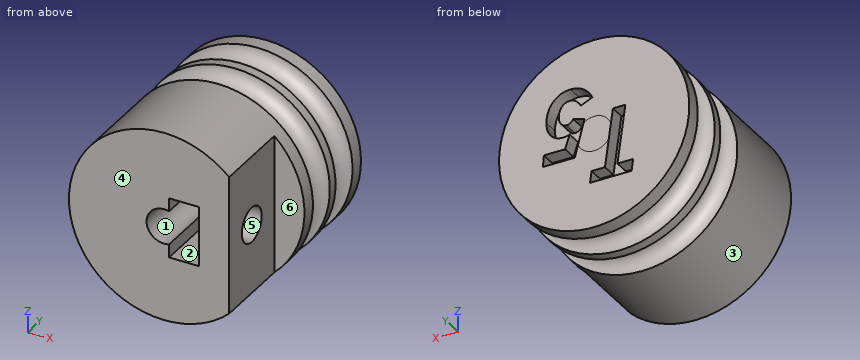
from build123d import *

# Parameters (mm, degrees)
SKETCH1_R               = 9.5
SKETCH1_R_2             = 1.75
BOSS_EXTRUDE1_DEPTH     = 18
SKETCH2_R               = 1.5
CUT_EXTRUDE1_DEPTH      = 23.461077445
CUT_EXTRUDE1_DEPTH_BACK = 23.461077445
SKETCH3_W               = 3
SKETCH3_H               = 8
SKETCH4_W               = 3
SKETCH4_H               = 6
CUT_EXTRUDE2_DEPTH      = 8
CUT_EXTRUDE3_REACH      = 27.889
SKETCH5_R               = 1.75
BOSS_EXTRUDE2_START     = -8.5
SKETCH6_R               = 1.75
BOSS_EXTRUDE2_DEPTH     = 8.5
CUT_EXTRUDE4_DEPTH      = 1.5


with BuildPart() as part:
    # Sketch1 → Boss-Extrude1 (new body)
    with BuildSketch(Plane(origin=(0, 0, 0), x_dir=(1, 0, 0), z_dir=(0, 1, 0))):
        with Locations(Location((0, 0, 0), (0, 0, 270))):
            Circle(SKETCH1_R)
        with Locations(Location((0, 0, 0), (0, 0, 270))):
            Circle(SKETCH1_R_2, mode=Mode.SUBTRACT)
    extrude(amount=BOSS_EXTRUDE1_DEPTH)

    # Sketch2 → Cut-Revolve1 (revolve, cut)
    with BuildSketch(Plane(origin=(0, 0, 0), x_dir=(0, 0, -1), z_dir=(1, 0, 0)), mode=Mode.PRIVATE) as cut_revolve1_sk:
        with Locations((-9.5, 15)):
            Circle(SKETCH2_R)
        with Locations((-9.5, 11)):
            Circle(SKETCH2_R)
    revolve(cut_revolve1_sk.sketch.rotate(Axis((0, 18, 0), (0, -1, 0)), 180), axis=Axis((0, 18, 0), (0, -1, 0)), mode=Mode.SUBTRACT)

    # Sketch3 → Cut-Extrude1 (cut, two sides: drawn at the far end of the back side and taken through both)
    with BuildSketch(Plane.XY.offset(-CUT_EXTRUDE1_DEPTH_BACK)):
        with Locations((8, 4)):
            Rectangle(SKETCH3_W, SKETCH3_H)
    extrude(amount=CUT_EXTRUDE1_DEPTH + CUT_EXTRUDE1_DEPTH_BACK, mode=Mode.SUBTRACT)

    # Sketch4 → Cut-Extrude2 (cut)
    with BuildSketch(Plane.XZ):
        with Locations((2, 0)):
            Rectangle(SKETCH4_W, SKETCH4_H)
    extrude(amount=-CUT_EXTRUDE2_DEPTH, mode=Mode.SUBTRACT)

    # Sketch5 → Cut-Extrude3 (cut, up to next)
    with BuildSketch(Plane(origin=(6.5, 0, 0), x_dir=(0, 0, -1), z_dir=(1, 0, 0)), mode=Mode.PRIVATE) as cut_extrude3_sk1:
        with Locations((0, 4)):
            Circle(SKETCH5_R)
    cut_extrude3_tool1 = extrude(cut_extrude3_sk1.sketch, amount=-CUT_EXTRUDE3_REACH, mode=Mode.PRIVATE) & part.part
    add(cut_extrude3_tool1.solids().sort_by_distance((6.5, 4, 0))[0], mode=Mode.SUBTRACT)

    # Sketch6 → Boss-Extrude2 (add)
    with BuildSketch(Plane(origin=(0, 18, 0), x_dir=(1, 0, 0), z_dir=(0, 1, 0)).offset(BOSS_EXTRUDE2_START)):
        with Locations(Location((0, 0, 0), (0, 0, 73.398450401))):
            Circle(SKETCH6_R)
    extrude(amount=BOSS_EXTRUDE2_DEPTH)

    # Sketch7 → Cut-Extrude4 (cut)
    with BuildSketch(Plane(origin=(0, 18, 0), x_dir=(1, 0, 0), z_dir=(0, 1, 0))):
        Polygon((-3.735416667, 4.879166667), (0.409722222, 4.879166667), (0.260894097, 3.732638889), (-1.078559028, 3.732638889), (-1.873687066, -2), (-3.118055556, -2), (-2.324305556, 3.732638889), (-3.893891059, 3.732638889), align=None)
        with BuildLine():
            Line((1.93063151, 1.879166667), (5.115277778, 1.879166667))
            Line((5.115277778, 1.879166667), (5.027083333, 0.732638889))
            Line((5.027083333, 0.732638889), (2.899392361, 0.732638889))
            Line((2.899392361, 0.732638889), (2.447395833, -0.634375))
            add(Edge.make_bspline(
                [(2.447395833, -0.634375), (2.496594075, -0.613896402), (2.595019861, -0.57292701), (2.749839769, -0.532892585), (2.908139813, -0.506658512), (3.015040488, -0.503615987), (3.068891059, -0.502083333)],
                knots=[0, 0, 0, 0, 0.998112439, 1.996819346, 2.990909824, 4, 4, 4, 4], degree=3))
            add(Edge.make_bspline(
                [(3.068891059, -0.502083333), (3.130977849, -0.503710927), (3.252390467, -0.506893737), (3.430147714, -0.530676662), (3.598897739, -0.570188022), (3.758037558, -0.627264893), (3.908251801, -0.698872885), (4.047892395, -0.787903157), (4.178629893, -0.892282921), (4.299407696, -1.011738133), (4.408795358, -1.145923516), (4.504121795, -1.293773987), (4.584127105, -1.455328827), (4.650907598, -1.628980167), (4.699239379, -1.817024844), (4.736887191, -2.016677617), (4.75910168, -2.230101729), (4.761345538, -2.376622611), (4.7625, -2.452007378)],
                knots=[0, 0, 0, 0, 1.020720285, 1.996049746, 2.943245614, 3.865445419, 4.770849874, 5.674014514, 6.582344456, 7.517049549, 8.461983903, 9.42367584, 10.403295435, 11.421749409, 12.477096939, 13.591170916, 14.760661157, 16, 16, 16, 16], degree=3))
            add(Edge.make_bspline(
                [(4.7625, -2.452007378), (4.760331263, -2.551305248), (4.756082769, -2.745827008), (4.724357481, -3.030366667), (4.670434408, -3.299932267), (4.596788587, -3.55576096), (4.497839346, -3.795403814), (4.381045078, -4.022055988), (4.240535383, -4.23285879), (4.079959926, -4.426863528), (3.90500901, -4.6032865), (3.715999291, -4.755276836), (3.51825895, -4.886229848), (3.309156679, -4.99341577), (3.088438962, -5.074038184), (2.858442877, -5.134443243), (2.617463381, -5.168719531), (2.453470724, -5.173806613), (2.370225694, -5.176388889)],
                knots=[0, 0, 0, 0, 1.173543811, 2.298939634, 3.378629864, 4.419763593, 5.440091566, 6.438176937, 7.429014836, 8.427971092, 9.41078854, 10.360474936, 11.289592146, 12.209863076, 13.130646371, 14.061665239, 15.016073429, 16, 16, 16, 16], degree=3))
            add(Edge.make_bspline(
                [(2.370225694, -5.176388889), (2.310933889, -5.175336104), (2.193952372, -5.173258982), (2.020726741, -5.156555087), (1.852671583, -5.127655453), (1.689527041, -5.086994539), (1.530531877, -5.038216677), (1.376964542, -4.976019014), (1.229625203, -4.900480546), (1.08541527, -4.817015387), (0.94797473, -4.720741688), (0.817898945, -4.612055658), (0.693643574, -4.493656656), (0.576265412, -4.363698122), (0.466116126, -4.222246293), (0.360964906, -4.071122574), (0.264514937, -3.907473589), (0.206115245, -3.793152274), (0.176388889, -3.734960938)],
                knots=[0, 0, 0, 0, 1.022859238, 2.018080294, 2.999190336, 3.962207893, 4.917235095, 5.866490093, 6.816373485, 7.771926692, 8.739336783, 9.707395925, 10.693964512, 11.698357727, 12.725720478, 13.785346591, 14.8727068, 16, 16, 16, 16], degree=3))
            Line((0.176388889, -3.734960938), (1.318782552, -3.225086806))
            add(Edge.make_bspline(
                [(1.318782552, -3.225086806), (1.366983822, -3.296490214), (1.457415836, -3.430452538), (1.598648511, -3.608942531), (1.738402882, -3.749836535), (1.87577747, -3.85858293), (2.016355711, -3.936444461), (2.160759687, -3.990581364), (2.311349194, -4.023320871), (2.413704476, -4.027668904), (2.46531033, -4.029861111)],
                knots=[0, 0, 0, 0, 1.407698414, 2.641030095, 3.71326683, 4.644229953, 5.494388505, 6.328183133, 7.157097367, 8, 8, 8, 8], degree=3))
            add(Edge.make_bspline(
                [(2.46531033, -4.029861111), (2.502597477, -4.028960648), (2.576241743, -4.027182182), (2.684301906, -4.008243163), (2.787874215, -3.97960222), (2.886816155, -3.939640908), (2.979376072, -3.886543817), (3.067364075, -3.822476619), (3.149686009, -3.745907333), (3.2282627, -3.660042601), (3.298101555, -3.562969472), (3.360585167, -3.458803462), (3.411342282, -3.34552927), (3.454177874, -3.225850289), (3.487464002, -3.098113353), (3.509883951, -2.962938195), (3.526380141, -2.82034566), (3.527303997, -2.722613415), (3.527777778, -2.67249349)],
                knots=[0, 0, 0, 0, 0.927075282, 1.831027126, 2.721359743, 3.598085148, 4.478603181, 5.370329063, 6.300781167, 7.271983059, 8.262041119, 9.271703604, 10.289679922, 11.345465186, 12.432354444, 13.569366541, 14.753500788, 16, 16, 16, 16], degree=3))
            add(Edge.make_bspline(
                [(3.527777778, -2.67249349), (3.525364071, -2.599249545), (3.520736664, -2.45883084), (3.479231749, -2.258812343), (3.4090829, -2.080955219), (3.310983371, -1.92926026), (3.194562907, -1.805997587), (3.06438106, -1.714608894), (2.920185823, -1.658694036), (2.819485773, -1.652001198), (2.768478733, -1.648611111)],
                knots=[0, 0, 0, 0, 1.239981349, 2.377214621, 3.442410989, 4.461421974, 5.419299017, 6.29797895, 7.137884662, 8, 8, 8, 8], degree=3))
            add(Edge.make_bspline(
                [(2.768478733, -1.648611111), (2.733962981, -1.650076188), (2.665766285, -1.652970908), (2.565430302, -1.671769102), (2.471751626, -1.70770096), (2.381470388, -1.752665642), (2.299031841, -1.814661474), (2.221082072, -1.888742142), (2.147448466, -1.975747239), (2.105339675, -2.041728663), (2.08359375, -2.075802951)],
                knots=[0, 0, 0, 0, 0.978206346, 1.932753505, 2.875607702, 3.812696253, 4.78098368, 5.784402359, 6.855815662, 8, 8, 8, 8], degree=3))
            Line((2.08359375, -2.075802951), (0.970138889, -1.745073785))
            Line((0.970138889, -1.745073785), (1.93063151, 1.879166667))
        make_face()
    extrude(amount=-CUT_EXTRUDE4_DEPTH, mode=Mode.SUBTRACT)


solid = part.part
Geometry check sheet. Reference: the model listing, model coordinates, mm. Face numbers are marked on the shaded views. A direction names the side the tool comes from. Give positions to 0.01 mm unless a question says otherwise; leave off trailing zeros. Loops run counter-clockwise (first coordinate to the right, second up) from the corner with the lowest first, then second, coordinate; pieces in that order, holes last. Notation, with made-up numbers: M -7.5,65 L 3.5,65 A30 cw 3.5,89 Z; hole C 78,29 d10. An arc over 180 degrees is marked long. Answer as a JSON object with one key per item and string values. Group by question number.
Item 1: Material ranges on L1, parallel to Z at x = 0, y = 3; L2, parallel to Y at x = 4.1, z = 0; L3, parallel to Y at x = 5.25, z = 7, recorded low to high.
Item 2: Gauge pin test, flat ends, axial feed: pin 1 (2.5 mm diameter, centred on y = 6, z = 1.5, fed in from +X); pin 2 (0.8 mm diameter, centred on x = -1.5, y = 17.5, fed in from +Z); pin 3 (1 mm diameter, centred on x = 3.5, y = 5, fed in from +Z). Record the tip position at first contact, or that the pin passes through.
Item 3: Sectioned sample at A-A on y = 7. Record the boundary of the cut face in (x, z).
Item 4: Sectioned sample at C-C on y = 4. Record the boundary of the cut face in (x, z).
Item 5: Mould release check, pull along X, two halves, no side actions. Record for the marked faces 1, 2, 3 and 4: pulls with the +X half, pulls with the -X half, needs draft (parallel to the pull), parting line crosses it, or undercut.
Item 6: Access from +Z, -Z, +X, -X, +Y, -Y to the whole of each face (thin tool, end or side, straight path). Record for the marked faces 5 and 6.
Item 7: Sectioned sample at D-D on z = 8. Give the number of separate pieces and of enclosed holes in the cut face, plus the area to 3 significant figures.
Findings below:
{
 "1": {"L1": "-9.5 to -1.75, 1.75 to 9.5", "L2": "0 to 2.25, 5.75 to 18", "L3": "0 to 9.7, 12.3 to 13.7, 16.3 to 18"},
 "2": {"pin 1": "x = 6.5", "pin 2": "z = 9.44", "pin 3": "z = 9.01"},
 "3": {"outline": "M 6.5,-6.93 L 6.5,6.93 A9.5 ccw long Z; hole M 0.5,-3 L 3.5,-3 L 3.5,3 L 0.5,3 L 0.5,1.68 A1.75 ccw long 0.5,-1.68 Z"},
 "4": {"outline": "M 0.5,-3 L 0.5,-1.68 A1.75 cw long 0.5,1.68 L 0.5,3 L 3.5,3 L 3.5,1.75 L 6.5,1.75 L 6.5,6.93 A9.5 ccw long 6.5,-6.93 L 6.5,-1.75 L 3.5,-1.75 L 3.5,-3 Z"},
 "5": {"face 1": "undercut", "face 2": "undercut", "face 3": "parting line crosses it", "face 4": "needs draft"},
 "6": {"face 5": "+X", "face 6": "+Z, -Z, +X, -Y"},
 "7": {"separate pieces": "3", "enclosed holes": "0", "area": "146 mm2"}
}
